Can you work these out from the model? Positions are in its coordinate system, mm. A direction names the side the tool comes from. Coordinates: 2 decimals unless noted, no trailing zeros. Order: outer loops, then holes, each group sorted by start corner. A loop starts at its lowest first (then second) coordinate and runs counter-clockwise, first axis right, second up. Notation, with made-up numbers: (73.25, 35.25) -> (97.25, 35.25) arc R28 ccw to (97.25, 74.25) -> close; hole circle Ø2 at (20.5, -1.75). An arc over 180 degrees is marked (long way). Answer in a Markdown table with one row per item. Add a question column.
1. Imagine slicing it at C-C on x = 195.5. Write out the boundary of the cut face in (y, z), plus the area to 3 significant figures.
2. We'd pull the mould along Y, two halves only. Please class faces 3 (the face through (0.867, -3.905, 3.662)), 4 (the face through (299.9, -4.3, 12)), 5 (the face through (154, -10, 5)): pulls with the +Y half, pulls with the -Y half, needs draft (parallel to the pull), parting line crosses it, or undercut.
3. Imagine slicing it at B-B on z = 7.5. Write out the boundary of the cut face in (x, y).
4. Will these pins go through, and if not, where does the flat tip stop? pin 1 (1.5 mm diameter, centred on x = 142.5, z = 9, fed in from +Y); pin 2 (2 mm diameter, centred on y = -2.5, z = 9.5, fed in from +X); pin 3 (13 mm diameter, centred on x = 300, y = 0, fed in from -Z).
5. Imagine slicing it at A-A on x = 0. Write out the boundary of the cut face in (y, z), plus the area to 3 significant figures.
6. On a 3-axis mill with a long thin cutter (end or side, diameter ignored), from which of +Z, -Z, +X, -X, +Y, -Y can I reach the whole of each face in a straight line? I mean faces 1 (the face through (304, 0, 6)), 2 (the face through (158, 10, 5)). Say none if no direction works.
7. If I drill on line 1 along Y through (x, z) = (300, 5); line 2 along Y through (x, z) = (250, 6); line 3 along Y through (x, z) = (0, 5.75), over which ranges is the centre line in solid material (lowest first)? Write a range as [from, to].
from build123d import *

# Parameters (mm, degrees)
SKETCH1_R             = 15
BOSS_EXTRUDE1_DEPTH   = 10
SKETCH1_R_2           = 10
BOSS_EXTRUDE1_2_DEPTH = 10
BOSS_EXTRUDE3_DEPTH   = 10
SKETCH13_R            = 4
CUT_EXTRUDE1_DEPTH    = 20
BOSS_EXTRUDE7_START   = 2.5
SKETCH14_R            = 15
SKETCH14_R_2          = 4
BOSS_EXTRUDE7_DEPTH   = 2.5
SKETCH15_R            = 4
BOSS_EXTRUDE8_DEPTH   = 2


with BuildPart() as part:
    # Sketch1 → Boss-Extrude1 (new body)
    with BuildSketch(Plane.XY):
        Circle(SKETCH1_R)
    extrude(amount=BOSS_EXTRUDE1_DEPTH)



with BuildPart() as body_2:
    # Sketch1 → Boss-Extrude1 2 (new body)
    with BuildSketch(Plane.XY):
        with Locations((300, 0)):
            Circle(SKETCH1_R_2)
    extrude(amount=BOSS_EXTRUDE1_2_DEPTH)


with BuildPart() as part_1:
    add(part.part)

    add(body_2.part)  # Boss-Extrude3 merges body 2
    # Sketch5 → Boss-Extrude3 (add)
    with BuildSketch(Plane.XY):
        with BuildLine():
            Line((300, 10), (11.180339887, 10))
            ThreePointArc((11.180339887, 10), (14.012585384, 5.352331347), (15, 0))
            ThreePointArc((15, 0), (14.012585384, -5.352331347), (11.180339887, -10))
            Line((11.180339887, -10), (300, -10))
            ThreePointArc((300, -10), (290, 0), (300, 10))
        make_face()
    extrude(amount=BOSS_EXTRUDE3_DEPTH)

    # Sketch13 → Cut-Extrude1 (cut)
    with BuildSketch(Plane(origin=(0, 0, 0), x_dir=(-1, 0, 0), z_dir=(0, 0, -1))):
        with Locations((-300, 0)):
            Circle(SKETCH13_R)
        Circle(SKETCH13_R)
    extrude(amount=-CUT_EXTRUDE1_DEPTH, mode=Mode.SUBTRACT)

    # Sketch14 → Boss-Extrude7 (add)
    with BuildSketch(Plane(origin=(0, 0, 0), x_dir=(-1, 0, 0), z_dir=(0, 0, -1)).offset(BOSS_EXTRUDE7_START)):
        Circle(SKETCH14_R)
        Circle(SKETCH14_R_2, mode=Mode.SUBTRACT)
    extrude(amount=-BOSS_EXTRUDE7_DEPTH)

    # Sketch15 → Boss-Extrude8 (add)
    with BuildSketch(Plane.XY.offset(10)):
        with BuildLine():
            ThreePointArc((300, 10), (290, 0), (300, -10))
            ThreePointArc((300, -10), (307.071067812, -7.071067812), (310, 0))
            ThreePointArc((310, 0), (307.071067812, 7.071067812), (300, 10))
        make_face()
        with Locations(Location((300, 0, 0), (0, 0, 180))):
            Circle(SKETCH15_R, mode=Mode.SUBTRACT)
    extrude(amount=BOSS_EXTRUDE8_DEPTH)


solid = part_1.part
Answers follow:
| question | item | result |
|---|---|---|
| 1 | outline | (-10, 0) -> (10, 0) -> (10, 10) -> (-10, 10) -> close |
| 1 | area | 200 mm² |
| 2 | face 3 | undercut |
| 2 | face 4 | needs draft |
| 2 | face 5 | pulls with the -Y half |
| 3 | outline | (11.18, -10) -> (300, -10) arc R10 ccw to (300, 10) -> (11.18, 10) arc R15 ccw (long way) to start; hole circle Ø8 at (0, 0); hole circle Ø8 at (300, 0) |
| 4 | pin 1 | stops at y = 10 |
| 4 | pin 2 | stops at x = 309.89 |
| 4 | pin 3 | stops at z = 0 |
| 5 | outline | (-15, -2.5) -> (-4, -2.5) -> (-4, 10) -> (-15, 10) -> close; (4, -2.5) -> (15, -2.5) -> (15, 10) -> (4, 10) -> close |
| 5 | area | 275 mm² |
| 6 | face 1 | +Z, -Z |
| 6 | face 2 | +Z, -Z, +X, +Y |
| 7 | line 1 | y = [-10, -4], [4, 10] |
| 7 | line 2 | y = [-10, 10] |
| 7 | line 3 | y = [-15, -4], [4, 15] |
